Geometry check sheet. Reference: the model listing, model coordinates, mm. Face numbers are marked on the shaded views. A direction names the side the tool comes from. Coordinates: 2 decimals unless noted, no trailing zeros. Write each loop counter-clockwise with the first axis right and the second up, starting at its lowest first coordinate (ties: lowest second). Pieces come first, ordered by that corner, then holes. Notation, with made-up numbers: (62, 65) -> (85, 65) arc R5 ccw to (85, 73) -> close; hole circle Ø9 at (62, 63). An arc over 180 degrees is marked (long way). Answer in a Markdown table with one row per item. Add a question column.
Q1. Thickness scan on line 1 (Y direction, x = 6, z = -6); line 2 (Z direction, x = 7, y = 94); line 3 (Z direction, x = 23, y = 58.5). Record the ranges inside material, lowest first.
Q2. Section check A-A, the plane x = 89. Record the boundary of the cut face in (y, z), and give its area (3 significant figures).
Q3. Section check D-D, the plane y = 6. Record the boundary of the cut face in (x, z), and give its area (3 significant figures).
Q4. Section check B-B, the plane z = -6. Record the boundary of the cut face in (x, y), and give its area (3 significant figures).
Q5. Gauge pin test, flat ends, axial feed: P1, Ø6, axis at y = 52, z = -74, coming from the -X side; P2, Ø3.5, axis at y = 88, z = -12, coming from the -X side; P3, Ø11, axis at x = 100, z = -3, coming from the -Y side. Record the tip position at first contact, or that the pin passes through.
Q6. Tool access check on the marked faces 1 and 2. Record the directions out of +Z, -Z, +X, -X, +Y, -Y that give a thin tool (end or side, any length) a straight path to the whole face; none if there is none.
Q7. Release check for a two-part mould opening along Z. For the marked faces 3, 4, 5 and 6 record: pulls with the +Z half, pulls with the -Z half, needs draft (parallel to the pull), parting line crosses it, or undercut.
Q8. Section check C-C, the plane y = 94. Record the boundary of the cut face in (x, z), and give its area (3 significant figures).
```python
from build123d import *

# Parameters (mm, degrees)
SKETCH2_W           = 130
SKETCH2_H           = 130
BOSS_EXTRUDE1_DEPTH = 100
SKETCH3_W           = 104
SKETCH3_H           = 74
CUT_EXTRUDE1_DEPTH  = 127
SKETCH4_W           = 10
SKETCH4_H           = 10
CUT_EXTRUDE3_DEPTH  = 105
SKETCH5_W           = 104
SKETCH5_H           = 10
CUT_EXTRUDE4_DEPTH  = 127
SKETCH6_W           = 10
SKETCH6_H           = 74
CUT_EXTRUDE5_DEPTH  = 127
SKETCH7_R           = 1.75
CUT_EXTRUDE6_DEPTH  = 20
SKETCH8_W           = 3
SKETCH8_H           = 3
CUT_EXTRUDE7_DEPTH  = 5
SKETCH9_W           = 85
SKETCH9_H           = 60
BOSS_EXTRUDE2_DEPTH = 15
SKETCH11_W          = 85
SKETCH11_H          = 6
BOSS_EXTRUDE5_DEPTH = 5
SKETCH12_W          = 85
SKETCH12_H          = 3
CUT_EXTRUDE9_DEPTH  = 4
SKETCH13_W          = 82
SKETCH13_H          = 57
CUT_EXTRUDE10_DEPTH = 15
SKETCH15_W          = 3
SKETCH15_H          = 3
BOSS_EXTRUDE7_DEPTH = 5
SKETCH16_W          = 82
SKETCH16_H          = 2
BOSS_EXTRUDE8_DEPTH = 57
SKETCH17_W          = 77
SKETCH17_H          = 47
CUT_EXTRUDE11_DEPTH = 10
SKETCH19_W          = 7
SKETCH19_H          = 2
SKETCH19_H_2        = 1
BOSS_EXTRUDE9_DEPTH = 1
SKETCH21_W          = 3
SKETCH21_H          = 3
CUT_EXTRUDE15_DEPTH = 5


with BuildPart() as part:
    # Sketch2 → Boss-Extrude1 (new body)
    with BuildSketch(Plane(origin=(0, 0, 0), x_dir=(1, 0, 0), z_dir=(0, 1, 0))):
        with Locations((65, 65)):
            Rectangle(SKETCH2_W, SKETCH2_H)
    extrude(amount=BOSS_EXTRUDE1_DEPTH)

    # Sketch3 → Cut-Extrude1 (cut)
    with BuildSketch(Plane.ZY):
        with Locations((-65, 50)):
            Rectangle(SKETCH3_W, SKETCH3_H)
    extrude(amount=-CUT_EXTRUDE1_DEPTH, mode=Mode.SUBTRACT)

    # Sketch4 → Cut-Extrude3 (cut)
    with BuildSketch(Plane(origin=(130, 0, 0), x_dir=(0, 0, -1), z_dir=(1, 0, 0))):
        with Locations((5, 95)):
            Rectangle(SKETCH4_W, SKETCH4_H)
        with Locations((125, 95)):
            Rectangle(SKETCH4_W, SKETCH4_H)
        with Locations((5, 5)):
            Rectangle(SKETCH4_W, SKETCH4_H)
        with Locations((125, 5)):
            Rectangle(SKETCH4_W, SKETCH4_H)
    extrude(amount=-CUT_EXTRUDE3_DEPTH, mode=Mode.SUBTRACT)

    # Sketch5 → Cut-Extrude4 (cut)
    with BuildSketch(Plane.ZY):
        with Locations((-65, 92)):
            Rectangle(SKETCH5_W, SKETCH5_H)
        with Locations((-65, 8)):
            Rectangle(SKETCH5_W, SKETCH5_H)
    extrude(amount=-CUT_EXTRUDE4_DEPTH, mode=Mode.SUBTRACT)

    # Sketch6 → Cut-Extrude5 (cut)
    with BuildSketch(Plane.ZY):
        with Locations((-122, 50)):
            Rectangle(SKETCH6_W, SKETCH6_H)
        with Locations((-8, 50)):
            Rectangle(SKETCH6_W, SKETCH6_H)
    extrude(amount=-CUT_EXTRUDE5_DEPTH, mode=Mode.SUBTRACT)

    # Sketch7 → Cut-Extrude6 (cut)
    with BuildSketch(Plane.ZY):
        with Locations((-124, 94)):
            Circle(SKETCH7_R)
        with Locations((-6, 94)):
            Circle(SKETCH7_R)
        with Locations((-124, 6)):
            Circle(SKETCH7_R)
        with Locations((-6, 6)):
            Circle(SKETCH7_R)
    extrude(amount=-CUT_EXTRUDE6_DEPTH, mode=Mode.SUBTRACT)

    # Sketch8 → Cut-Extrude7 (cut)
    with BuildSketch(Plane.ZY):
        with Locations((-118.5, 88.5)):
            Rectangle(SKETCH8_W, SKETCH8_H)
        with Locations((-11.5, 88.5)):
            Rectangle(SKETCH8_W, SKETCH8_H)
        with Locations((-118.5, 11.5)):
            Rectangle(SKETCH8_W, SKETCH8_H)
        with Locations((-11.5, 11.5)):
            Rectangle(SKETCH8_W, SKETCH8_H)
    extrude(amount=-CUT_EXTRUDE7_DEPTH, mode=Mode.SUBTRACT)

    # Sketch9 → Boss-Extrude2 (add)
    with BuildSketch(Plane(origin=(0, 3, 0), x_dir=(1, 0, 0), z_dir=(0, 1, 0))):
        with Locations((42.5, 87)):
            Rectangle(SKETCH9_W, SKETCH9_H)
    extrude(amount=BOSS_EXTRUDE2_DEPTH)

    # Sketch11 → Boss-Extrude5 (add)
    with BuildSketch(Plane(origin=(0, 13, 0), x_dir=(1, 0, 0), z_dir=(0, 1, 0))):
        with Locations((42.5, 120)):
            Rectangle(SKETCH11_W, SKETCH11_H)
    extrude(amount=BOSS_EXTRUDE5_DEPTH)

    # Sketch12 → Cut-Extrude9 (cut)
    with BuildSketch(Plane(origin=(0, 18, 0), x_dir=(1, 0, 0), z_dir=(0, 1, 0))):
        with Locations((42.5, 121.5)):
            Rectangle(SKETCH12_W, SKETCH12_H)
    extrude(amount=-CUT_EXTRUDE9_DEPTH, mode=Mode.SUBTRACT)

    # Sketch13 → Cut-Extrude10 (cut)
    with BuildSketch(Plane(origin=(0, 18, 0), x_dir=(1, 0, 0), z_dir=(0, 1, 0))):
        with Locations((41, 88.5)):
            Rectangle(SKETCH13_W, SKETCH13_H)
    extrude(amount=-CUT_EXTRUDE10_DEPTH, mode=Mode.SUBTRACT)

    # Sketch15 → Boss-Extrude7 (add)
    with BuildSketch(Plane.ZY.offset(-5)):
        with Locations((-118.5, 11.5)):
            Rectangle(SKETCH15_W, SKETCH15_H)
    extrude(amount=BOSS_EXTRUDE7_DEPTH)

    # Sketch16 → Boss-Extrude8 (add)
    with BuildSketch(Plane(origin=(0, 0, -60), x_dir=(-1, 0, 0), z_dir=(0, 0, -1))):
        with Locations((-41, 17)):
            Rectangle(SKETCH16_W, SKETCH16_H)
        with Locations((-41, 12)):
            Rectangle(SKETCH16_W, SKETCH16_H)
    extrude(amount=BOSS_EXTRUDE8_DEPTH)

    # Sketch17 → Cut-Extrude11 (cut)
    with BuildSketch(Plane(origin=(0, 18, 0), x_dir=(1, 0, 0), z_dir=(0, 1, 0))):
        with Locations((38.5, 88.5)):
            Rectangle(SKETCH17_W, SKETCH17_H)
    extrude(amount=-CUT_EXTRUDE11_DEPTH, mode=Mode.SUBTRACT)

    # Sketch19 → Boss-Extrude9 (add)
    with BuildSketch(Plane.XY.offset(-117)):
        with Locations((3.5, 10)):
            Rectangle(SKETCH19_W, SKETCH19_H)
        with Locations((3.5, 13.5)):
            Rectangle(SKETCH19_W, SKETCH19_H_2)
    extrude(amount=BOSS_EXTRUDE9_DEPTH)

    # Sketch21 → Cut-Extrude15 (cut)
    with BuildSketch(Plane.ZY):
        with Locations((-118.5, 11.5)):
            Rectangle(SKETCH21_W, SKETCH21_H)
    extrude(amount=-CUT_EXTRUDE15_DEPTH, mode=Mode.SUBTRACT)


solid = part.part
```
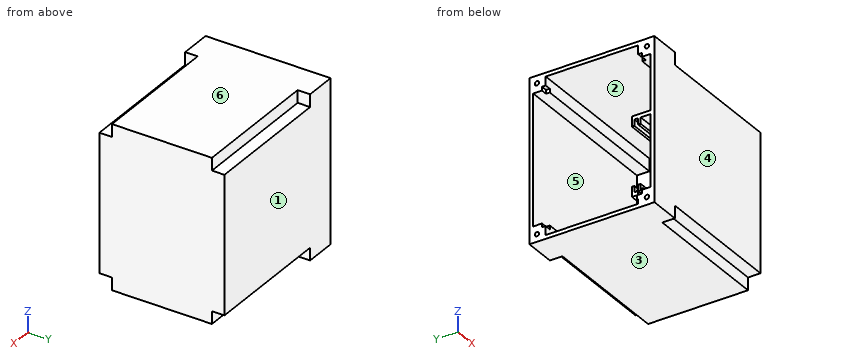
Calculated:
| question | item | result |
|---|---|---|
| 1 | line 1 | y = 0 to 4.25, 7.75 to 13, 87 to 92.25, 95.75 to 100 |
| 1 | line 2 | z = -130 to -125.75, -122.25 to -117, -13 to -7.75, -4.25 to 0 |
| 1 | line 3 | z = -130 to -127, -3 to 0 |
| 2 | outline | (0, -120) -> (10, -120) -> (10, -130) -> (90, -130) -> (90, -120) -> (100, -120) -> (100, -10) -> (90, -10) -> (90, 0) -> (10, 0) -> (10, -10) -> (0, -10) -> close; hole (3, -117) -> (13, -117) -> (13, -127) -> (87, -127) -> (87, -117) -> (97, -117) -> (97, -13) -> (87, -13) -> (87, -3) -> (13, -3) -> (13, -13) -> (3, -13) -> close |
| 2 | area | 1,340 mm² |
| 3 | outline | (0, -130) -> (25, -130) -> (25, -120) -> (130, -120) -> (130, -10) -> (25, -10) -> (25, 0) -> (0, 0) -> (0, -4.25) -> (20, -4.25) -> (20, -7.75) -> (0, -7.75) -> (0, -13) -> (127, -13) -> (127, -117) -> (85, -117) -> (85, -57) -> (0, -57) -> (0, -60) -> (82, -60) -> (82, -117) -> (0, -117) -> (0, -122.25) -> (20, -122.25) -> (20, -125.75) -> (0, -125.75) -> close |
| 3 | area | 1,880 mm² |
| 4 | outline | (0, 0) -> (25, 0) -> (25, 10) -> (130, 10) -> (130, 90) -> (25, 90) -> (25, 100) -> (0, 100) -> (0, 95.75) -> (20, 95.75) -> (20, 92.25) -> (0, 92.25) -> (0, 87) -> (127, 87) -> (127, 13) -> (0, 13) -> (0, 7.75) -> (20, 7.75) -> (20, 4.25) -> (0, 4.25) -> close |
| 4 | area | 1,360 mm² |
| 5 | P1 | stops at x = 127 |
| 5 | P2 | stops at x = 5 |
| 5 | P3 | stops at y = 10 |
| 6 | face 1 | +Z, -Z, +X, -X, +Y |
| 6 | face 2 | -X |
| 7 | face 3 | pulls with the -Z half |
| 7 | face 4 | needs draft |
| 7 | face 5 | undercut |
| 7 | face 6 | pulls with the +Z half |
| 8 | outline | (0, -130) -> (25, -130) -> (25, -120) -> (130, -120) -> (130, -10) -> (25, -10) -> (25, 0) -> (0, 0) -> (0, -4.25) -> (20, -4.25) -> (20, -7.75) -> (0, -7.75) -> (0, -13) -> (127, -13) -> (127, -117) -> (0, -117) -> (0, -122.25) -> (20, -122.25) -> (20, -125.75) -> (0, -125.75) -> close |
| 8 | area | 1,450 mm² |
